from build123d import *

# Parameters (mm, degrees)
BOSS_EXTRUDE1_DEPTH               = 25.4889
BOSS_EXTRUDE2_DEPTH               = 10.9982
TAP_DRILL_FOR_M12X1_75_TAP1_D     = 10.2
TAP_DRILL_FOR_M12X1_75_TAP1_DEPTH = 19.05
TAP_DRILL_FOR_M12X1_75_TAP1_TIP   = 3.064389157
TAP_DRILL_FOR_M12X1_75_TAP2_D     = 10.2
TAP_DRILL_FOR_M12X1_75_TAP2_DEPTH = 19.05
TAP_DRILL_FOR_M12X1_75_TAP2_TIP   = 3.064389157


with BuildPart() as part:
    # Sketch1 → Boss-Extrude1 (new body)
    with BuildSketch(Plane.XY):
        with BuildLine():
            Line((-24.8285, -38.0873), (24.8285, -38.0873))
            Line((24.8285, -38.0873), (24.8285, -24.3713))
            Line((24.8285, -24.3713), (-8.5471, -24.3713))
            ThreePointArc((-8.5471, -24.3713), (-13.5255, -19.3929), (-8.5471, -14.4145))
            Line((-8.5471, -14.4145), (24.8285, -14.4145))
            Line((24.8285, -14.4145), (24.8285, 38.0873))
            Line((24.8285, 38.0873), (-24.8285, 38.0873))
            Line((-24.8285, 38.0873), (-24.8285, 24.3713))
            Line((-24.8285, 24.3713), (8.5471, 24.3713))
            ThreePointArc((8.5471, 24.3713), (13.5255, 19.3929), (8.5471, 14.4145))
            Line((8.5471, 14.4145), (-24.8285, 14.4145))
            Line((-24.8285, 14.4145), (-24.8285, -38.0873))
        make_face()
    extrude(amount=BOSS_EXTRUDE1_DEPTH)

    # Sketch2 → Boss-Extrude2 (add)
    with BuildSketch(Plane(origin=(24.8285, 0, 0), x_dir=(0, 0, -1), z_dir=(1, 0, 0))):
        Polygon((-11.700587864, 3.150816299), (-13.873781444, -2.815734603), (-9.79319358, -7.681050902), (-3.539412136, -6.579816299), (-1.366218556, -0.613265397), (-5.44680642, 4.252050902), align=None)
    extrude(amount=BOSS_EXTRUDE2_DEPTH)

    # Tap Drill for M12x1.75 Tap1
    with Locations(Plane(origin=(0, 38.0873, 0), x_dir=(1, 0, 0), z_dir=(0, 1, 0))):
        with Locations((0, -12.74445)):
            Hole(TAP_DRILL_FOR_M12X1_75_TAP1_D / 2, depth=TAP_DRILL_FOR_M12X1_75_TAP1_DEPTH)
            with Locations((0, 0, -(TAP_DRILL_FOR_M12X1_75_TAP1_DEPTH + TAP_DRILL_FOR_M12X1_75_TAP1_TIP / 2))):  # 118° drill point
                Cone(0, TAP_DRILL_FOR_M12X1_75_TAP1_D / 2, TAP_DRILL_FOR_M12X1_75_TAP1_TIP, mode=Mode.SUBTRACT)

    # Tap Drill for M12x1.75 Tap2
    with Locations(Plane(origin=(0, -38.0873, 0), x_dir=(-1, 0, 0), z_dir=(0, -1, 0))):
        with Locations((0, -12.74445)):
            Hole(TAP_DRILL_FOR_M12X1_75_TAP2_D / 2, depth=TAP_DRILL_FOR_M12X1_75_TAP2_DEPTH)
            with Locations((0, 0, -(TAP_DRILL_FOR_M12X1_75_TAP2_DEPTH + TAP_DRILL_FOR_M12X1_75_TAP2_TIP / 2))):  # 118° drill point
                Cone(0, TAP_DRILL_FOR_M12X1_75_TAP2_D / 2, TAP_DRILL_FOR_M12X1_75_TAP2_TIP, mode=Mode.SUBTRACT)


solid = part.part
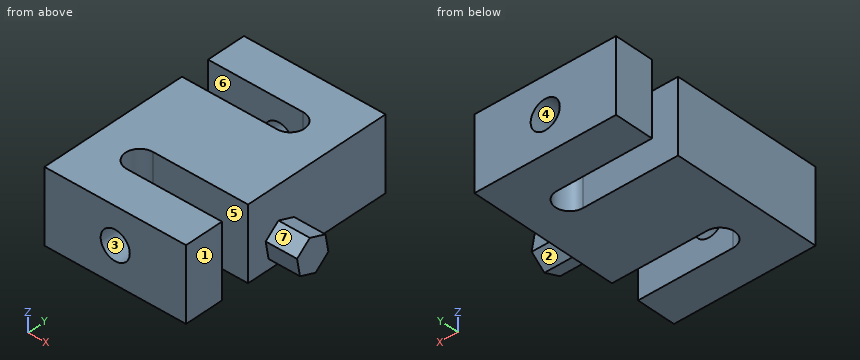
Part model, mm, in its own coordinate system. Face numbers are marked on the shaded views. A direction names the side the tool comes from. Coordinates: 2 decimals unless noted, no trailing zeros. Loops run counter-clockwise (first coordinate to the right, second up) from the corner with the lowest first, then second, coordinate; pieces in that order, holes last. Notation, with made-up numbers: (5, -3) - (62, -3) arc R19 ccw to (62, 32) - close; hole circle Ø3 at (25.5, 54). An arc over 180 degrees is marked (long way). Write each question's results on one line, items separated by ' | '. Start each with the question number.
Q1. Which spindle directions (+Z, -Z, +X, -X, +Y, -Y) get a long thin tool onto all of the face, cutting with end or side? Do the marked faces 4, 5, 6 and 7. Say none if no direction does.
Q2. Slice it at B-B on z = 8.75. Give the cut face in (x, y), and give its area (3 significant figures).
Q3. Slice it at C-C on x = 19. Give the cut face in (y, z).
Q4. Slice it at D-D on y = -4.5. Give the cut face in (x, z).
Q5. Slice it at A-A on x = 0. Give the cut face in (y, z).
Q6. Probe line 1 along Y through (x, z) = (-8.5, 22.75); line 2 along Y through (x, z) = (21, 24.25); line 3 along Y through (x, z) = (-19, 6.5). List the from-to ranges inside material, lowest first.
Q7. Two-plate mould, pull along Z, no slides. Class the marked faces 1, 2 and 3: +Z half, -Z half, draft (parallel to the pull), parting line (faces both ways), or undercut.
Q8. Drop flat-ended pins along their axis: pin 1 Ø12.5 at (y, z) = (21.5, 12.5) entering from +X; pin 2 Ø6 at (x, z) = (0, 12.74) entering from +Y; pin 3 Ø6 at (x, z) = (0, 12.74) entering from -Y. Give the stop position or say it passes through.
Answer:
1) face 4: +Y | face 5: +Z, -Z, +X | face 6: +Z, -Z, -X | face 7: +Z, +X, -Y
2) outline: (-24.83, -38.09) - (-3.17, -38.09) - (-3.17, -24.37) - (-8.55, -24.37) arc R4.98 cw to (-8.55, -14.41) - (24.83, -14.41) - (24.83, -7.5) - (35.83, -7.5) - (35.83, 3.67) - (24.83, 3.67) - (24.83, 38.09) - (3.17, 38.09) - (3.17, 24.37) - (8.55, 24.37) arc R4.98 cw to (8.55, 14.41) - (-24.83, 14.41) - close; (-24.83, 24.37) - (-3.17, 24.37) - (-3.17, 38.09) - (-24.83, 38.09) - close; (3.17, -38.09) - (24.83, -38.09) - (24.83, -24.37) - (3.17, -24.37) - close | area: 2,990 mm2
3) outline: (-38.09, 0) - (-24.37, 0) - (-24.37, 25.49) - (-38.09, 25.49) - close; (-14.41, 0) - (38.09, 0) - (38.09, 25.49) - (-14.41, 25.49) - close
4) outline: (-24.83, 0) - (24.83, 0) - (24.83, 2.78) - (35.83, 2.78) - (35.83, 12.46) - (24.83, 12.46) - (24.83, 25.49) - (-24.83, 25.49) - close
5) outline: (-38.09, 0) - (-24.37, 0) - (-24.37, 7.64) - (-38.09, 7.64) - close; (-38.09, 17.84) - (-24.37, 17.84) - (-24.37, 25.49) - (-38.09, 25.49) - close; (-14.41, 0) - (14.41, 0) - (14.41, 25.49) - (-14.41, 25.49) - close; (24.37, 0) - (38.09, 0) - (38.09, 7.64) - (24.37, 7.64) - close; (24.37, 17.84) - (38.09, 17.84) - (38.09, 25.49) - (24.37, 25.49) - close
6) line 1: y = -38.09 to -24.37, -14.41 to 14.41, 24.37 to 38.09 | line 2: y = -38.09 to -24.37, -14.41 to 38.09 | line 3: y = -38.09 to 14.41, 24.37 to 38.09
7) face 1: draft | face 2: -Z half | face 3: undercut
8) pin 1: stops at x = 24.83 | pin 2: stops at y = 14.41 | pin 3: stops at y = -14.41
